Work out the finished part from the listing and answer in its coordinate system (mm). Round coordinates to 2 decimals unless told otherwise and drop trailing zeros. Write each loop counter-clockwise with the first axis right and the second up, starting at its lowest first coordinate (ties: lowest second). Pieces come first, ordered by that corner, then holes. Notation, with made-up numbers: M 70.25,31.5 L 100.25,31.5 A33 ccw 100.25,63.5 Z; hole C 59,33.25 d4. An arc over 180 degrees is marked long. One line per item, written item: value. Start each with the question number.
Q1. Find section A-A (z = -83.5). Write down the section's boundary in (x, y), and give its area (3 significant figures).
Q2. Given pin 1 Ø2.5 at (x, y) = (-14, 4.5) entering from -Z; pin 2 Ø3 at (x, z) = (14.5, -122) entering from +Y, each flat-ended and moving along its own axis, determine where each tip first touches the part or whether it passes through.
Q3. Consider probe 1 along Y at (x, z) = (13, 87); probe 2 along X at (y, z) = (16, 90); probe 3 along X at (y, z) = (8.5, -21.5). Determine where each line is inside the solid, lowest interval first.
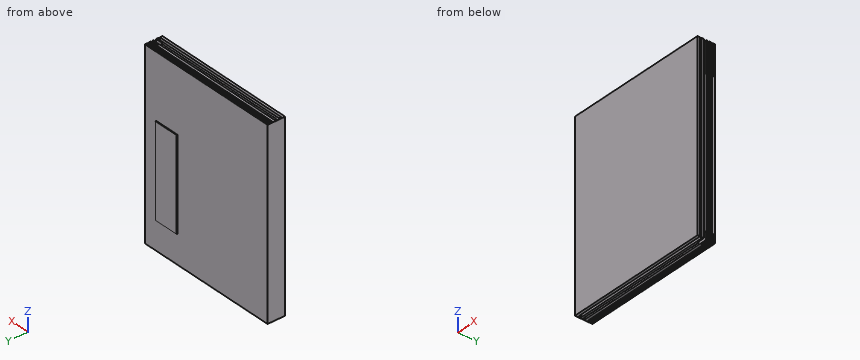
from build123d import *

# Parameters (mm, degrees)
SKETCH_1_W          = 190
SKETCH_1_H          = 240
EXTRUDE_1_DEPTH     = 23
SKETCH_2_W          = 244.953894582
SKETCH_2_H          = 1.92087839
SKETCH_2_W_2        = 245.721377573
SKETCH_2_H_2        = 1.683754508
SKETCH_2_W_3        = 244.530855974
SKETCH_2_H_3        = 3.204341319
SKETCH_2_W_4        = 243.54031242
SKETCH_2_H_4        = 1.944573874
CUT_EXTRUDE_1_DEPTH = 10
SKETCH_3_W          = 187.993982421
SKETCH_3_H          = 1.571683417
SKETCH_3_W_2        = 186.752481484
SKETCH_3_H_2        = 1.663815778
SKETCH_3_H_3        = 2.618871028
SKETCH_3_H_4        = 3.346100481
CUT_EXTRUDE_2_DEPTH = 40
SKETCH_10_W         = 32.883336007
SKETCH_10_H         = 119.476120829
EXTRUDE_2_DEPTH     = 1


with BuildPart() as part:
    # 草图1 → 凸台-拉伸1 (new body)
    with BuildSketch(Plane(origin=(0, 0, 0), x_dir=(1, 0, 0), z_dir=(0, 1, 0))):
        with Locations((0, 5)):
            Rectangle(SKETCH_1_W, SKETCH_1_H)
    extrude(amount=EXTRUDE_1_DEPTH)

    # 草图2 → 切除-拉伸1 (cut)
    with BuildSketch(Plane(origin=(95, 0, 0), x_dir=(0, 0, -1), z_dir=(1, 0, 0))):
        with Locations((6.062274081, 18.228253569)):
            Rectangle(SKETCH_2_W, SKETCH_2_H)
        with Locations((6.148753652, 14.520829351)):
            Rectangle(SKETCH_2_W_2, SKETCH_2_H_2)
        with Locations((5.553492852, 9.89782934)):
            Rectangle(SKETCH_2_W_3, SKETCH_2_H_3)
        with Locations((5.313676242, 4.397346814)):
            Rectangle(SKETCH_2_W_4, SKETCH_2_H_4)
    extrude(amount=-CUT_EXTRUDE_1_DEPTH, mode=Mode.SUBTRACT)

    # 草图3 → 切除-拉伸2 (cut)
    with BuildSketch(Plane.XY.offset(115)):
        with Locations((1.003008789, 20.115789148)):
            Rectangle(SKETCH_3_W, SKETCH_3_H)
        with Locations((0.382258321, 16.316351191)):
            Rectangle(SKETCH_3_W_2, SKETCH_3_H_2)
        with Locations((0.382258321, 10.748217394)):
            Rectangle(SKETCH_3_W_2, SKETCH_3_H_3)
        with Locations((0.382258321, 5.041481802)):
            Rectangle(SKETCH_3_W_2, SKETCH_3_H_4)
    cut_extrude_2 = extrude(amount=-CUT_EXTRUDE_2_DEPTH, mode=Mode.SUBTRACT)

    # 镜向3: 切除-拉伸2 across plane
    add(cut_extrude_2.mirror(Plane.XY.offset(-20)), mode=Mode.SUBTRACT)

    # 草图10 → 凸台-拉伸2 (add)
    with BuildSketch(Plane(origin=(0, 23, 0), x_dir=(1, 0, 0), z_dir=(0, 1, 0))):
        with Locations((61.016856815, 28.018335206)):
            Rectangle(SKETCH_10_W, SKETCH_10_H)
    extrude(amount=EXTRUDE_2_DEPTH)


solid = part.part
The answers:
1. outline: M -95,0 L 95,0 L 95,3.43 L 85,3.43 L 85,5.37 L 95,5.37 L 95,8.3 L 85,8.3 L 85,11.5 L 95,11.5 L 95,13.68 L 85,13.68 L 85,15.36 L 95,15.36 L 95,17.27 L 85,17.27 L 85,19.19 L 95,19.19 L 95,23 L 77.46,23 L 77.46,24 L 44.58,24 L 44.58,23 L -95,23 Z
1. area: 4,320 mm2
2. pin 1: z = -125
2. pin 2: y = 23
3. probe 1: 0 to 3.37, 6.71 to 9.44, 12.06 to 15.48, 17.15 to 19.33, 20.9 to 23
3. probe 2: -95 to -92.99, 93.76 to 95
3. probe 3: -95 to 85
